The model under review builds one solid part; all positions refer to its coordinate system, in mm. A direction names the side the tool comes from. Give positions to 0.01 mm unless a question says otherwise; leave off trailing zeros. Order: outer loops, then holes, each group sorted by start corner. A loop starts at its lowest first (then second) coordinate and runs counter-clockwise, first axis right, second up.
```python
from build123d import *

# Parameters (mm, degrees)
BOSS_EXTRUDE1_DEPTH      = 38.1
BOSS_EXTRUDE1_DEPTH_BACK = 38.1
SKETCH1_W                = 4.5
SKETCH1_H                = 8.12
SKETCH2_R                = 4
CUT_EXTRUDE1_DEPTH       = 55.4
SKETCH3_R                = 6.5
CUT_EXTRUDE2_DEPTH       = 8.2
CUT_EXTRUDE3_START       = 19.05
SKETCH4_W                = 20
SKETCH4_H                = 15
CUT_EXTRUDE3_DEPTH       = 10


with BuildPart() as part:
    # Sketch1 → Boss-Extrude1 (new, two sides: drawn at the far end of the back side and taken through both)
    with BuildSketch(Plane.XY.offset(-BOSS_EXTRUDE1_DEPTH_BACK)):
        with BuildLine():
            ThreePointArc((7.62, 16.748), (6.912893219, 15.040893219), (8.62, 15.748))
            Line((8.62, 15.748), (19.05, 15.748))
            Line((19.05, 15.748), (19.05, 0))
            Line((19.05, 0), (0, 0))
            Line((0, 0), (0, 25.4))
            Line((0, 25.4), (7.62, 25.4))
            Line((7.62, 25.4), (7.62, 16.748))
        make_face()
        with Locations((21.3, 7.874)):
            Rectangle(SKETCH1_W, SKETCH1_H)
    extrude(amount=BOSS_EXTRUDE1_DEPTH + BOSS_EXTRUDE1_DEPTH_BACK)

    # Sketch2 → Cut-Extrude1 (cut)
    with BuildSketch(Plane(origin=(0, 0, 0), x_dir=(0, 0, -1), z_dir=(1, 0, 0))):
        with Locations(Location((-19.05, 8, 0), (0, 0, 100.422660027))):
            Circle(SKETCH2_R)
        with Locations(Location((19.05, 8, 0), (0, 0, 100.422660027))):
            Circle(SKETCH2_R)
    extrude(amount=CUT_EXTRUDE1_DEPTH, mode=Mode.SUBTRACT)

    # Sketch3 → Cut-Extrude2 (cut)
    with BuildSketch(Plane(origin=(0, 0, 0), x_dir=(0, 0, -1), z_dir=(1, 0, 0))):
        with Locations((-19.05, 8)):
            Circle(SKETCH3_R)
        with Locations((19.05, 8)):
            Circle(SKETCH3_R)
    extrude(amount=CUT_EXTRUDE2_DEPTH, mode=Mode.SUBTRACT)

    # Sketch4 → Cut-Extrude3 (cut)
    with BuildSketch(Plane(origin=(0, 0, 0), x_dir=(0, 0, -1), z_dir=(1, 0, 0)).offset(CUT_EXTRUDE3_START)):
        with Locations((-19.05, 8)):
            Rectangle(SKETCH4_W, SKETCH4_H)
        with Locations((19.05, 8)):
            Rectangle(SKETCH4_W, SKETCH4_H)
    extrude(amount=CUT_EXTRUDE3_DEPTH, mode=Mode.SUBTRACT)


solid = part.part
```
1. Take a section at C-C (z = 31.5). Write out the cut boundary in (x, y).
2. Draft analysis for pull direction Y (two halves, no side actions). For faces 6 (the flat face through (8.2, 5, 22)), 7 (the cylindrical face through (4.043, 14.445, 19.896)), 8 (the flat face through (21, 8, -29.05)), 9 (the flat face through (14, 15.748, -1)), state which applies: pulls with the +Y half, pulls with the -Y half, needs draft (parallel to the pull), parting line crosses it, or undercut.
3. Take a section at B-B (y = 8). Write out the cut boundary in (x, z), and give its area (3 significant figures).
4. Take a section at D-D (x = 3). Write out the cut boundary in (y, z).
5. To check wall thickness, follow line 1 (Z direction, x = 11.75, y = 8); line 2 (Z direction, x = 20.25, y = 10.25); line 3 (Y direction, x = 2.75, z = -19). State the ranges of each line that lie inside material, in increasing order.
6. Take a section at A-A (z = -19.05). Write out the cut boundary in (x, y), and give its area (3 significant figures).
7. For faces 1 (the flat face through (23.55, 8, 0)), 2 (the flat face through (8.2, 5, -16)), 3 (the flat face through (21, 3.814, 34)), 4 (the flat face through (21, 11.934, 0)), 5 (the flat face through (9, 10, 38.1)), list the 3-axis set-ups (+Z, -Z, +X, -X, +Y, -Y) from which the entire face can be reached by the end or side of a thin tool; tool diameter is ignored.
8. Insertion check: pin 1 (5 mm diameter, centred on x = 20.5, z = -35, fed in from +Y); pin 2 (1.3 mm diameter, centred on x = 22, z = -34.5, fed in from -Y); pin 3 (11.5 mm diameter, centred on y = 8, z = -19.05, fed in from -X). Each pin has a flat end and moves straight along its axis. Give the tip position at first contact, or say it passes through.
Answer:
1. outline: (0, 0) - (19.05, 0) - (19.05, 3.81) - (23.55, 3.81) - (23.55, 11.93) - (19.05, 11.93) - (19.05, 15.75) - (8.62, 15.75) arc R1 cw (long way) to (7.62, 16.75) - (7.62, 25.4) - (0, 25.4) - close
2. face 6: undercut
2. face 7: undercut
2. face 8: needs draft
2. face 9: pulls with the +Y half
3. outline: (0, -38.1) - (23.55, -38.1) - (23.55, -29.05) - (19.05, -29.05) - (19.05, -23.05) - (8.2, -23.05) - (8.2, -25.55) - (0, -25.55) - close; (0, -12.55) - (8.2, -12.55) - (8.2, -15.05) - (19.05, -15.05) - (19.05, -9.05) - (23.55, -9.05) - (23.55, 9.05) - (19.05, 9.05) - (19.05, 15.05) - (8.2, 15.05) - (8.2, 12.55) - (0, 12.55) - close; (0, 25.55) - (8.2, 25.55) - (8.2, 23.05) - (19.05, 23.05) - (19.05, 29.05) - (23.55, 29.05) - (23.55, 38.1) - (0, 38.1) - close
3. area: 1,230 mm2
4. outline: (0, -38.1) - (25.4, -38.1) - (25.4, 38.1) - (0, 38.1) - close; hole circle Ø13 at (8, -19.05); hole circle Ø13 at (8, 19.05)
5. line 1: z = -38.1 to -23.05, -15.05 to 15.05, 23.05 to 38.1
5. line 2: z = -38.1 to -29.05, -9.05 to 9.05, 29.05 to 38.1
5. line 3: y = 0 to 1.5, 14.5 to 25.4
6. outline: (0, 0) - (19.05, 0) - (19.05, 4) - (8.2, 4) - (8.2, 1.5) - (0, 1.5) - close; (0, 14.5) - (8.2, 14.5) - (8.2, 12) - (19.05, 12) - (19.05, 15.75) - (8.62, 15.75) arc R1 cw (long way) to (7.62, 16.75) - (7.62, 25.4) - (0, 25.4) - close
6. area: 178 mm2
7. face 1: +Z, -Z, +X, +Y, -Y
7. face 2: -X
7. face 3: +Z, -Z, +X, -Y
7. face 4: +Z, -Z, +X, +Y
7. face 5: +Z, +X, -X, +Y, -Y
8. pin 1: stops at y = 15.75
8. pin 2: stops at y = 3.81
8. pin 3: stops at x = 8.2
